Input: part model. Units: mm. Frame: model coordinates. Face numbers are marked on the shaded views. Round coordinates to 2 decimals unless told otherwise and drop trailing zeros. Loops run counter-clockwise (first coordinate to the right, second up) from the corner with the lowest first, then second, coordinate; pieces in that order, holes last. Notation, with made-up numbers: (62.25, 59) - (120.25, 59) arc R16 ccw to (120.25, 82) - close; hole circle Ø8 at (0, -15). An arc over 180 degrees is marked (long way). Write each question's results on one line, items separated by ' | '.
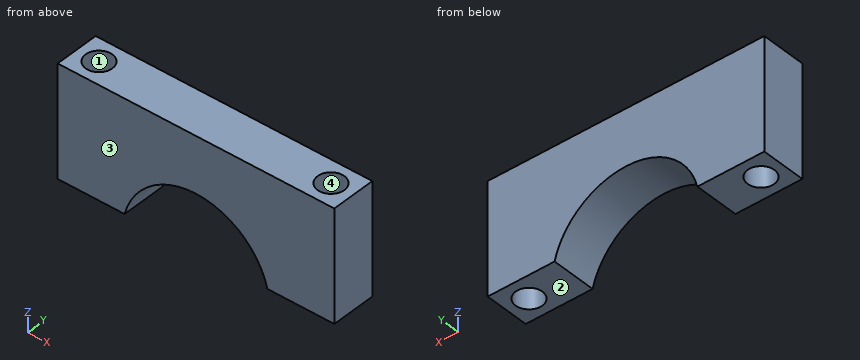
from build123d import *

# Parameters (mm, degrees)
BOSS_EXTRUDE1_DEPTH = 10
SKETCH2_R           = 3
CUT_EXTRUDE1_DEPTH  = 27


with BuildPart() as part:
    # Sketch1 → Boss-Extrude1 (new body)
    with BuildSketch(Plane(origin=(0, 0, 0), x_dir=(1, 0, 0), z_dir=(0, 1, 0))):
        with BuildLine():
            Line((-16.007810594, -4), (-31.007810594, -4))
            Line((-31.007810594, -4), (-31.007810594, -29))
            Line((-31.007810594, -29), (-22, -29))
            Line((-22, -29), (22, -29))
            Line((22, -29), (31.007810594, -29))
            Line((31.007810594, -29), (31.007810594, -4))
            Line((31.007810594, -4), (16.007810594, -4))
            ThreePointArc((16.007810594, -4), (0, -16.5), (-16.007810594, -4))
        make_face()
    extrude(amount=BOSS_EXTRUDE1_DEPTH)

    # Sketch2 → Cut-Extrude1 (cut)
    with BuildSketch(Plane(origin=(0, 0, 4), x_dir=(-1, 0, 0), z_dir=(0, 0, -1))):
        with Locations((-26.007810594, 5)):
            Circle(SKETCH2_R)
        with Locations((26.007810594, 5)):
            Circle(SKETCH2_R)
    extrude(amount=-CUT_EXTRUDE1_DEPTH, mode=Mode.SUBTRACT)


solid = part.part
1. Section query B-B, the plane y = 5. Output: boundary loops of the cut face in (x, z), plus the area to 3 significant figures.
Answer:
outline: (-31.01, 4) - (-29.01, 4) - (-29.01, 29) - (-31.01, 29) - close; (-23.01, 4) - (-16.01, 4) arc R16.5 cw to (16.01, 4) - (23.01, 4) - (23.01, 29) - (-23.01, 29) - close; (29.01, 4) - (31.01, 4) - (31.01, 29) - (29.01, 29) - close | area: 953 mm^2
2. Mould query, pull axis Y, two halves, no side actions, for the marked faces 1, 2, 3 and 4. Classes: pulls with the +Y half, pulls with the -Y half, needs draft (parallel to the pull), parting line crosses it, or undercut.
Answer:
face 1: undercut | face 2: needs draft | face 3: pulls with the -Y half | face 4: undercut
3. Contact query for a flat-ended pin moving along its axis: pin 1 (3.5 mm diameter, centred on x = 26.01, y = 5, fed in from +Z). Output: stop coordinate, or through.
Answer:
pin 1: through
4. Section query D-D, the plane x = -10.5. Output: boundary loops of the cut face in (y, z), plus the area to 3 significant figures.
Answer:
outline: (0, 12.73) - (10, 12.73) - (10, 29) - (0, 29) - close | area: 163 mm^2
5. Line query: line 1 (X direction, y = 7.5, z = 27.5); line 2 (X direction, y = 6, z = 21.75); line 3 (X direction, y = 6.5, z = 11.5). Output: solid intervals per line, ascending. Write a range as [from, to].
Answer:
line 1: [-31.01, -27.67], [-24.35, 24.35], [27.67, 31.01] | line 2: [-31.01, -28.84], [-23.18, 23.18], [28.84, 31.01] | line 3: [-31.01, -28.61], [-23.41, -11.83], [11.83, 23.41], [28.61, 31.01]
6. Section query C-C, the plane y = 9. Output: boundary loops of the cut face in (x, z).
Answer:
outline: (-31.01, 4) - (-16.01, 4) arc R16.5 cw to (16.01, 4) - (31.01, 4) - (31.01, 29) - (-31.01, 29) - close
7. Section query A-A, the plane z = 11.5. Output: boundary loops of the cut face in (x, y).
Answer:
outline: (-31.01, 0) - (-11.83, 0) - (-11.83, 10) - (-31.01, 10) - close; (11.83, 0) - (31.01, 0) - (31.01, 10) - (11.83, 10) - close; hole circle Ø6 at (-26.01, 5); hole circle Ø6 at (26.01, 5)
